from build123d import *

# Parameters (mm, degrees)
BOSS_EXTRUDE4_DEPTH      = 24
SHELL1_T                 = -2
SKETCH9_R                = 1
CUT_EXTRUDE1_DEPTH       = 22
SKETCH6_R                = 1
BOSS_EXTRUDE5_DEPTH      = 4
BOSS_EXTRUDE6_START      = -4
SKETCH8_R                = 1
BOSS_EXTRUDE6_DEPTH      = 4
BOSS_EXTRUDE7_START      = -24
BOSS_EXTRUDE7_DEPTH      = 24
FILLET1_R                = 1
FILLET2_R                = 1.5
SKETCH12_R               = 0.5
BOSS_EXTRUDE8_DEPTH      = 24
CUT_EXTRUDE3_DEPTH       = 11
CUT_EXTRUDE4_DEPTH       = 11
BOSS_EXTRUDE9_DEPTH      = 2.5
BOSS_EXTRUDE9_DEPTH_BACK = 4.5
CUT_EXTRUDE5_DEPTH       = 0.747850193


with BuildPart() as part:
    # Sketch5 → Boss-Extrude4 (new body)
    with BuildSketch(Plane(origin=(0, 0, 0), x_dir=(1, 0, 0), z_dir=(0, 1, 0))):
        with BuildLine():
            Line((16.679736529, -62.588474268), (23.082859001, -66.493602001))
            ThreePointArc((23.082859001, -66.493602001), (44.985866831, -20.069862482), (44.587534446, 31.259921018))
            Line((44.587534446, 31.259921018), (54.42418125, 33.060026475))
            Line((54.42418125, 33.060026475), (53.884149613, 36.011020517))
            Line((53.884149613, 36.011020517), (37.98404912, 33.101303594))
            ThreePointArc((37.98404912, 33.101303594), (38.745638884, 14.245000299), (26.08183659, 0.253277589))
            ThreePointArc((26.08183659, 0.253277589), (27.736010667, -32.118438365), (16.679736529, -62.588474268))
        make_face()
    extrude(amount=BOSS_EXTRUDE4_DEPTH)

    # Shell1
    shell1_openings = [part.faces().sort_by_distance(p)[0] for p in [
        (27.736010667, 12, 32.118438365),
    ]]
    offset(amount=SHELL1_T, openings=shell1_openings, kind=Kind.INTERSECTION)

    # Sketch9 → Cut-Extrude1 (cut)
    with BuildSketch(Plane(origin=(0, 22, 0), x_dir=(-1, 0, 0), z_dir=(0, -1, 0))):
        with Locations(Location((-33, 0, 0), (0, 0, 90))):
            Circle(SKETCH9_R)
        Polygon((-18.802526646, -7.044160924), (-31.283524546, -4.66015009), (-31.283524546, 0.878893836), (-33, 1.78957842), (-36.853763417, 0.878893836), (-41.704444312, 7.207877481), (-44.902710544, 14.373324664), (-42.809869411, 29.924231084), (-24.798121137, 26.483784785), align=None)
    extrude(amount=CUT_EXTRUDE1_DEPTH, mode=Mode.SUBTRACT)

    # Sketch6 → Boss-Extrude5 (add)
    with BuildSketch(Plane(origin=(0, 24, 0), x_dir=(1, 0, 0), z_dir=(0, 1, 0))):
        with Locations(Location((33, 0, 0), (0, 0, 90))):
            Circle(SKETCH6_R)
    extrude(amount=-BOSS_EXTRUDE5_DEPTH)

    # Sketch8 → Boss-Extrude6 (add)
    with BuildSketch(Plane(origin=(0, 0, 0), x_dir=(-1, 0, 0), z_dir=(0, -1, 0)).offset(BOSS_EXTRUDE6_START)):
        with Locations(Location((-33, 0, 0), (0, 0, 270))):
            Circle(SKETCH8_R)
    extrude(amount=BOSS_EXTRUDE6_DEPTH)

    # Sketch11 → Boss-Extrude7 (add)
    with BuildSketch(Plane(origin=(0, 24, 0), x_dir=(1, 0, 0), z_dir=(0, 1, 0)).offset(BOSS_EXTRUDE7_START)):
        with BuildLine():
            Line((16.679736529, -62.588474268), (23.082859001, -66.493602001))
            ThreePointArc((23.082859001, -66.493602001), (28.946672892, -58.305690928), (34.074211637, -49.637672267))
            Line((34.074211637, -49.637672267), (24.945218618, -44.308006728))
            ThreePointArc((24.945218618, -44.308006728), (21.37536937, -53.70275106), (16.679736529, -62.588474268))
        make_face()
    extrude(amount=BOSS_EXTRUDE7_DEPTH)

    # Fillet1
    fillet1_edges = [part.edges().sort_by_distance(p)[0] for p in [
        (23.082859001, 12, 66.493602001),
        (16.679736529, 12, 62.588474268),
    ]]
    fillet(fillet1_edges, radius=FILLET1_R)

    # Fillet2
    fillet2_edges = [part.edges().sort_by_distance(p)[0] for p in [
        (39.36869634, 11, -29.266928363),
        (37.98404912, 12, -33.101303594),
        (53.884149613, 12, -36.011020517),
        (54.42418125, 12, -33.060026475),
        (44.587534446, 12, -31.259921018),
    ]]
    fillet(fillet2_edges, radius=FILLET2_R - 0.0001)  # a hair under: the kernel refuses the full size

    # Sketch12 → Boss-Extrude8 (add)
    with BuildSketch(Plane(origin=(0, 0, 0), x_dir=(1, 0, 0), z_dir=(0, 1, 0))):
        with BuildLine():
            Line((18.715601118, -63.830104629), (10.728103117, -74.664444727))
            ThreePointArc((10.728103117, -74.664444727), (10.299090631, -76.000345168), (11.504530989, -75.282295557))
            Line((11.504530989, -75.282295557), (19.996225612, -64.611130176))
            Line((19.996225612, -64.611130176), (18.715601118, -63.830104629))
        make_face()
        with Locations(Location((10.766093359, -75.413481937, 0), (0, 0, 270))):
            Circle(SKETCH12_R, mode=Mode.SUBTRACT)
    extrude(amount=BOSS_EXTRUDE8_DEPTH)

    # Sketch13 → Cut-Extrude3 (cut)
    with BuildSketch(Plane(origin=(0, 0, 0), x_dir=(1, 0, 0), z_dir=(0, 1, 0))):
        Polygon((19.996225612, -64.611130176), (24.885458438, -67.592968924), (14.482058763, -80.670297518), (6.551415536, -74.361237485), (17.528327491, -63.106011785), align=None)
    extrude(amount=CUT_EXTRUDE3_DEPTH, mode=Mode.SUBTRACT)

    # Sketch14 → Cut-Extrude4 (cut)
    with BuildSketch(Plane(origin=(0, 24, 0), x_dir=(1, 0, 0), z_dir=(0, 1, 0))):
        Polygon((19.996225612, -64.611130176), (15.918276164, -82.297397679), (4.930036713, -72.505157079), (18.705017469, -63.823649888), align=None)
    extrude(amount=-CUT_EXTRUDE4_DEPTH, mode=Mode.SUBTRACT)

    # Sketch15 → Boss-Extrude9 (add, two sides: drawn at the far end of the back side and taken through both)
    with BuildSketch(Plane(origin=(0, 13, 0), x_dir=(1, 0, 0), z_dir=(0, 1, 0)).offset(-BOSS_EXTRUDE9_DEPTH_BACK)):
        Polygon((19.018790552, -64.015013394), (17.840516782, -65.653708569), (18.447701563, -66.090293672), (19.659102799, -64.405526167), align=None)
    extrude(amount=BOSS_EXTRUDE9_DEPTH + BOSS_EXTRUDE9_DEPTH_BACK)

    # Sketch16 → Cut-Extrude5 (cut)
    with BuildSketch(Plane(origin=(43.486111653, 0, 31.267892586), x_dir=(0.5837868426462293, 0, -0.8119069665627625), z_dir=(0.8119069665627625, 0, 0.5837868426462293))):
        Polygon((-42.889644405, 13), (-40.814569828, 15.5), (-42.889644405, 15.5), align=None)
        Polygon((-42.889644405, 11), (-40.814569828, 8.5), (-42.889644405, 8.5), align=None)
    extrude(amount=-CUT_EXTRUDE5_DEPTH, mode=Mode.SUBTRACT)


solid = part.part
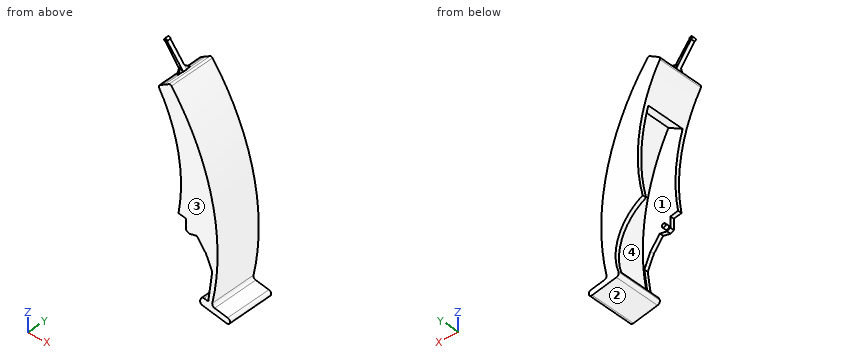
Check sheet for the modelled part. Datum: model origin and axes. Units: mm. Face numbers are marked on the shaded views. Round coordinates to 2 decimals unless told otherwise and drop trailing zeros. Loops run counter-clockwise (first coordinate to the right, second up) from the corner with the lowest first, then second, coordinate; pieces in that order, holes last. Notation, with made-up numbers: (-30.75, 39) -> (-9.75, 39) arc R29 ccw to (-9.75, 77) -> close; hole circle Ø9 at (-2, -5). An arc over 180 degrees is marked (long way). Put each result on its own line as item: value. Start each with the question number.
1. Gauge pin test, flat ends, axial feed: pin 1 (11 mm diameter, centred on x = 14, z = 70.5, fed in from -Y); pin 2 (6 mm diameter, centred on y = 13.5, z = -4, fed in from +X); pin 3 (2 mm diameter, centred on y = 1, z = 1, fed in from -X). Record the tip position at first contact, or that the pin passes through.
2. Draft check along Z on the marked faces 1, 2, 3 and 4. Enter one of: +Z half, -Z half, draft (parallel to the pull), parting line (faces both ways), or undercut.
3. Section check C-C (z = 29). Enter the section's corners in (x, y).
4. Scan lines: probe 1 along X at (y, z) = (20.75, -3); probe 2 along Z at (x, y) = (26.5, 20); probe 3 along X at (y, z) = (16.25, 16). Record each from-to range of solid material in increasing order.
5. Section check A-A (z = 2). Enter the section's corners in (x, y).
6. Section check D-D (z = 55). Enter the section's corners in (x, y).
Findings:
1. pin 1: stops at y = 11
1. pin 2: stops at x = 47.68
1. pin 3: stops at x = 31.28
2. face 1: undercut
2. face 2: -Z half
2. face 3: draft
2. face 4: undercut
3. outline: (28.14, 0) -> (42.64, 0) -> (42.64, 24) -> (28.14, 24) -> (28.14, 22) -> (40.55, 22) -> (40.55, 2) -> (28.14, 2) -> close
4. probe 1: x = 45.67 to 47.67
4. probe 2: z = 45.22 to 61.91
4. probe 3: x = 43.77 to 45.8
5. outline: (26.62, 22) -> (45.48, 22) -> (45.48, 2) -> (31.28, 2) -> (31.28, 0) -> (47.48, 0) -> (47.48, 24) -> (26.62, 24) -> close
6. outline: (20.78, 0) -> (31.02, 0) -> (31.02, 24) -> (20.78, 24) -> close
